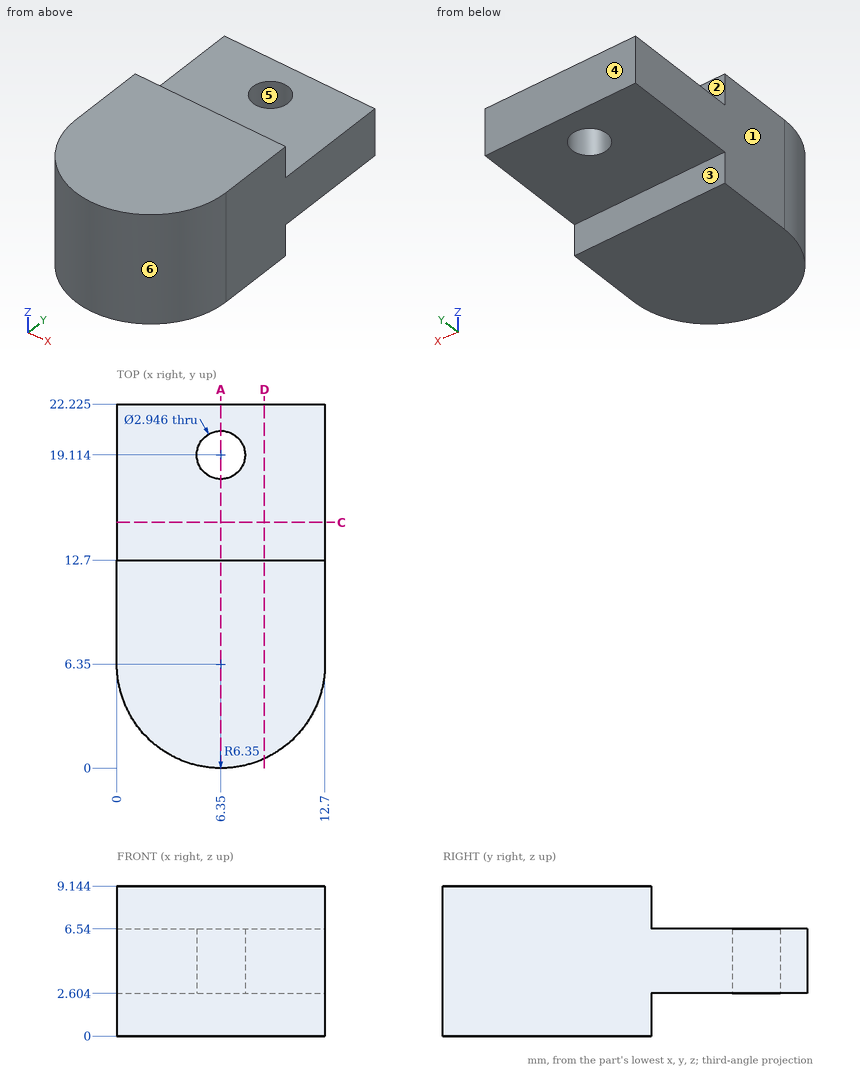
Input: dimensioned drawing with shaded views. Units: mm. Origin: part minimum x, y, z. A direction names the side the tool comes from. Coordinates: 2 decimals unless noted, no trailing zeros. Order: outer loops, then holes, each group sorted by start corner. A loop starts at its lowest first (then second) coordinate and runs counter-clockwise, first axis right, second up.
Item 1: Section query D-D (x = 9). Output: boundary loops of the cut face in (y, z) (1 decimal), then the cut area to 3 significant figures.
Answer:
outline: (0.6, 0) - (12.7, 0) - (12.7, 2.6) - (22.2, 2.6) - (22.2, 6.5) - (12.7, 6.5) - (12.7, 9.1) - (0.6, 9.1) - close
area: 148 mm2
Item 2: Material intervals for line 1 along Y through (x, z) = (6.35, 4.6) (1 decimal); line 2 along X through (y, z) = (19, 4.5); line 3 along Z through (x, y) = (9, 18.5), sorted ascending.
Answer:
line 1: y = 0 to 17.6, 20.6 to 22.2
line 2: x = 0 to 4.88, 7.82 to 12.7
line 3: z = 2.6 to 6.54
Item 3: Section query A-A (x = 6.35). Output: boundary loops of the cut face in (y, z) (1 decimal).
Answer:
outline: (0, 0) - (12.7, 0) - (12.7, 2.6) - (17.6, 2.6) - (17.6, 6.5) - (12.7, 6.5) - (12.7, 9.1) - (0, 9.1) - close; (20.6, 2.6) - (22.2, 2.6) - (22.2, 6.5) - (20.6, 6.5) - close
Item 4: Contact query for flat-ended pins moving along their axis: P1, Ø0.8, axis at x = 5, z = 8, coming from the +Y side; P2, Ø2.5, axis at x = 6.35, y = 19.11, coming from the -Z side; P3, Ø3, axis at x = 4, y = 19.5, coming from the -Z side. Output: stop coordinate, or through.
Answer:
P1: stops at y = 12.7
P2: passes through
P3: stops at z = 2.6
Item 5: Draft query along Y for the marked faces 4, 5 and 6. Return one class per face: released by +Y, released by -Y, zero draft, split by the parting line, or undercut.
Answer:
face 4: released by +Y
face 5: undercut
face 6: released by -Y
Item 6: Access query for the marked faces 1, 2 and 3. Directions: +Z, -Z, +X, -X, +Y, -Y. A direction counts if a zero-diameter tool reaches every point of the face in a straight line with its end or side. Return the directions, or none.
Answer:
face 1: +Z, -Z, -X, +Y, -Y
face 2: +Z, +X, -X, +Y
face 3: -Z, +X, -X, +Y
Item 7: Section query C-C (y = 15). Output: boundary loops of the cut face in (x, z), then the cut area to 3 significant figures.
Answer:
outline: (0, 2.6) - (12.7, 2.6) - (12.7, 6.54) - (0, 6.54) - close
area: 50.0 mm2
